Geometry check sheet. Reference: the model listing, model coordinates, mm. A direction names the side the tool comes from. Round coordinates to 2 decimals unless told otherwise and drop trailing zeros. Write each loop counter-clockwise with the first axis right and the second up, starting at its lowest first coordinate (ties: lowest second). Pieces come first, ordered by that corner, then holes. Notation, with made-up numbers: (74.25, 52) -> (118.25, 52) arc R12 ccw to (118.25, 63) -> close; hole circle Ø7 at (-18, 21.5). An arc over 180 degrees is marked (long way). Use a Markdown table: item, result.
```python
from build123d import *

# Parameters (mm, degrees)
SKETCH2_W           = 127
SKETCH2_H           = 152.4
BOSS_EXTRUDE2_DEPTH = 5.334
SKETCH3_W           = 127
SKETCH3_H           = 65.278
CUT_EXTRUDE1_DEPTH  = 100.333486579
CAVITY1_START       = -76.163714286
CAVITY1_OUTLINE_W   = 5.334
CAVITY1_OUTLINE_H   = 5.334
CAVITY1_DEPTH       = 29.028571429
CAVITY1_START_2     = -18.106571429
CAVITY1_2_OUTLINE_W = 5.334
CAVITY1_2_OUTLINE_H = 5.334
CAVITY1_2_DEPTH     = 23.694571429


# Read off the part's stored shape, not the designer's step: Cavity1
with BuildPart() as part:
    # Sketch2 → Boss-Extrude2 (new body)
    with BuildSketch(Plane.XY):
        Rectangle(SKETCH2_W, SKETCH2_H)
    extrude(amount=BOSS_EXTRUDE2_DEPTH)

    # Sketch3 → Cut-Extrude1 (cut, through all)
    with BuildSketch(Plane.XY.offset(5.334)):
        with Locations((0, 43.561)):
            Rectangle(SKETCH3_W, SKETCH3_H)
    extrude(amount=-CUT_EXTRUDE1_DEPTH, mode=Mode.SUBTRACT)

    # Cavity1 outline → Cavity1 (cut)
    with BuildSketch(Plane(origin=(0, 0, 0), x_dir=(1, 0, 0), z_dir=(0, 1, 0)).offset(CAVITY1_START)):
        with Locations((60.833, -2.667)):
            Rectangle(CAVITY1_OUTLINE_W, CAVITY1_OUTLINE_H)
        with Locations((-60.833, -2.667)):
            Rectangle(CAVITY1_OUTLINE_W, CAVITY1_OUTLINE_H)
    extrude(amount=CAVITY1_DEPTH, mode=Mode.SUBTRACT)

    # Cavity1 2 outline → Cavity1 2 (cut)
    with BuildSketch(Plane(origin=(0, 0, 0), x_dir=(1, 0, 0), z_dir=(0, 1, 0)).offset(CAVITY1_START_2)):
        with Locations((60.833, -2.667)):
            Rectangle(CAVITY1_2_OUTLINE_W, CAVITY1_2_OUTLINE_H)
        with Locations((-60.833, -2.667)):
            Rectangle(CAVITY1_2_OUTLINE_W, CAVITY1_2_OUTLINE_H)
    extrude(amount=CAVITY1_2_DEPTH, mode=Mode.SUBTRACT)


solid = part.part
```
(1) Gauge pin test, flat ends, axial feed: pin 1 Ø1 at (y, z) = (-17, 1) entering from +X; pin 2 Ø1.6 at (y, z) = (-62, 3) entering from -X. Record the tip position at first contact, or that the pin passes through.
A:
| item | result |
|---|---|
| pin 1 | stops at x = 58.17 |
| pin 2 | stops at x = -58.17 |
(2) Release check for a two-part mould opening along Y. For faces 4 (the face through (-1, -32, 5.334)), 5 (the face through (-1, 10.922, 3)), 6 (the face through (-58.166, -62, 3)) record: +Y half, -Y half, draft (parallel to the pull), parting line (faces both ways), or undercut.
A:
| item | result |
|---|---|
| face 4 | draft |
| face 5 | +Y half |
| face 6 | undercut |
(3) Section check B-B on y = -63. Record the cut outline in (x, z).
A:
| item | result |
|---|---|
| outline | (-58.17, 0) -> (58.17, 0) -> (58.17, 5.33) -> (-58.17, 5.33) -> close |
(4) Thickness scan on line 1 (X direction, y = -56.5, z = 2.55). Record the ranges inside material, lowest first.
A:
| item | result |
|---|---|
| line 1 | x = -58.17 to 58.17 |
(5) Access from +Z, -Z, +X, -X, +Y, -Y to the whole of each face (thin tool, end or side, straight path). Record for faces 1 (the face through (-61, -18.107, 3)), 2 (the face through (58.166, -6, 3)), 3 (the face through (-63.5, 8, 3)).
A:
| item | result |
|---|---|
| face 1 | +Z, -Z, -X |
| face 2 | +Z, -Z, +X |
| face 3 | +Z, -Z, -X, +Y, -Y |
